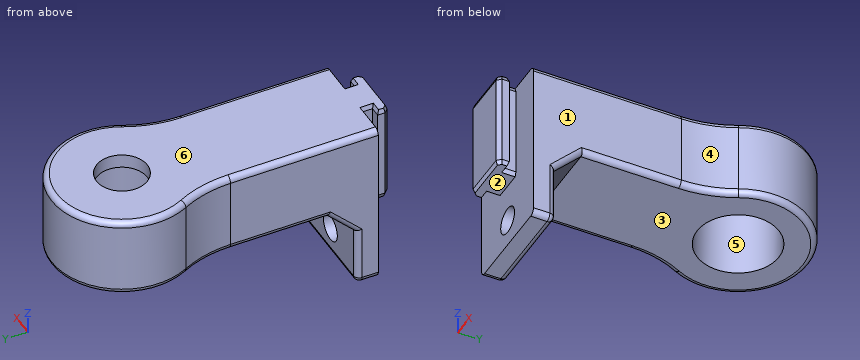
```python
from build123d import *
from OCP.BRepFilletAPI import BRepFilletAPI_MakeChamfer

# Parameters (mm, degrees)
SKETCH_1_R          = 4.5
EXTRUDE_1_DEPTH     = 2.5
EXTRUDE_START       = -12
SKETCH_1_13_R       = 7.25
SKETCH_1_13_R_2     = 4.5
EXTRUDE_5_DEPTH     = 12
EXTRUDE_START_2     = -7.5
EXTRUDE_2_DEPTH     = 20
EXTRUDE_3_DEPTH     = 15.5
SKETCH_4_R          = 2.4
CUT_EXTRUDE_3_DEPTH = 58.989223137
CUT_EXTRUDE_5_DEPTH = 0.1
CHAMFER_3_SIZE      = 0.8
CHAMFER_3_SIZE2     = 0.291176187
CHAMFER_4_SIZE      = 5
FILLET_1_R          = 1


with BuildPart() as part:
    # 草图1 → 凸台-拉伸1 (new body)
    with BuildSketch(Plane.XY):
        with BuildLine():
            Line((2.9, 10), (9, 10))
            Line((9, 10), (9, 36.328599249))
            ThreePointArc((9, 36.328599249), (9.545912037, 40.969554058), (11.153846154, 45.357153557))
            ThreePointArc((11.153846154, 45.357153557), (0, 63.5), (-11.153846154, 45.357153557))
            ThreePointArc((-11.153846154, 45.357153557), (-9.545912037, 40.969554058), (-9, 36.328599249))
            Line((-9, 36.328599249), (-9, 10))
            Line((-9, 10), (-2.9, 10))
            Line((-2.9, 10), (-2.9, 8))
            Line((-2.9, 8), (-4.7, 8))
            Line((-4.7, 8), (-4.7, 6.7))
            Line((-4.7, 6.7), (-4, 6))
            Line((-4, 6), (4, 6))
            Line((4, 6), (4.7, 6.7))
            Line((4.7, 6.7), (4.7, 8))
            Line((4.7, 8), (2.9, 8))
            Line((2.9, 8), (2.9, 10))
        make_face()
        with Locations((0, 51)):
            Circle(SKETCH_1_R, mode=Mode.SUBTRACT)
    extrude(amount=EXTRUDE_1_DEPTH)

    # 草图1<13> → 凸台-拉伸5 (add)
    # profile 1 of 4: a face of its own
    with BuildSketch(Plane.XY.offset(EXTRUDE_START)):
        Polygon((2.9, 10), (9, 10), (9, 14), (-9, 14), (-9, 10), (-2.9, 10), align=None)
    # profile 2 of 4: a face of its own
    with BuildSketch(Plane.XY.offset(EXTRUDE_START)):
        Polygon((2.9, 8), (2.9, 10), (-2.9, 10), (-2.9, 8), (-4.7, 8), (-4.7, 6.7), (-4, 6), (4, 6), (4.7, 6.7), (4.7, 8), align=None)
    # profile 3 of 4: a face of its own
    with BuildSketch(Plane.XY.offset(EXTRUDE_START)):
        with BuildLine():
            Line((-9, 14), (9, 14))
            Line((9, 14), (9, 36.328599249))
            ThreePointArc((9, 36.328599249), (9.545912037, 40.969554058), (11.153846154, 45.357153557))
            ThreePointArc((11.153846154, 45.357153557), (0, 63.5), (-11.153846154, 45.357153557))
            ThreePointArc((-11.153846154, 45.357153557), (-9.545912037, 40.969554058), (-9, 36.328599249))
            Line((-9, 36.328599249), (-9, 14))
        make_face()
        with Locations((0, 51)):
            Circle(SKETCH_1_13_R, mode=Mode.SUBTRACT)
    # profile 4 of 4: a face of its own
    with BuildSketch(Plane.XY.offset(EXTRUDE_START)):
        with Locations((0, 51)):
            Circle(SKETCH_1_13_R_2)
    extrude(amount=EXTRUDE_5_DEPTH)


with BuildPart() as extrude_5_kept_piece:
    # of the separate pieces the step leaves, the one the design keeps (extrude_5_pieces_kept)
    add(part.part.solids().sort_by_distance((2.9, 10, 2.5))[0])

    # 草图1<10> → 凸台-拉伸2 (add)
    with BuildSketch(Plane.XY.offset(EXTRUDE_START_2)):
        Polygon((2.9, 10), (9, 10), (9, 14), (-9, 14), (-9, 10), (-2.9, 10), align=None)
    extrude(amount=-EXTRUDE_2_DEPTH)

    # 草图1<11> → 凸台-拉伸3 (add)
    with BuildSketch(Plane.XY):
        Polygon((2.9, 8), (4.7, 8), (4.7, 6.7), (4, 6), (-4, 6), (-4.7, 6.7), (-4.7, 8), (-2.9, 8), (-2.9, 10), (2.9, 10), align=None)
    extrude(amount=-EXTRUDE_3_DEPTH)

    # 草图4 → 切除-拉伸3 (cut, through all)
    with BuildSketch(Plane(origin=(0, 14, 0), x_dir=(1, 0, 0), z_dir=(0, 1, 0))):
        with Locations(Location((0, 22.5, 0), (0, 0, 270))):
            Circle(SKETCH_4_R)
    extrude(amount=-CUT_EXTRUDE_3_DEPTH, mode=Mode.SUBTRACT)

    # 草图7 → 切除-拉伸5 (cut)
    with BuildSketch(Plane.XZ.offset(-10)):
        Polygon((2.9, 2.5), (9, 2.5), (9, -27.5), (-9, -27.5), (-9, 2.5), (-2.9, 2.5), (-2.9, -15.5), (2.9, -15.5), align=None)
    extrude(amount=-CUT_EXTRUDE_5_DEPTH, mode=Mode.SUBTRACT)

    # 倒角3: one chamfer whose edges measure the first distance from different faces: ONE call of the kernel's chamfer builder (chamfer() names one face for all edges)
    chamfer_3_edges_1 = [extrude_5_kept_piece.edges().sort_by_distance(p)[0] for p in [
        (2.9, 9.05, -15.5),
        (2.9, 9.05, 2.5),
    ]]
    chamfer_3_side_1 = [extrude_5_kept_piece.faces().sort_by_distance(p)[0] for p in [
        (2.9, 9.05, -6.5),
    ]]
    chamfer_3_edges_2 = [extrude_5_kept_piece.edges().sort_by_distance(p)[0] for p in [
        (4.7, 7.35, -15.5),
        (4.7, 7.35, 2.5),
    ]]
    chamfer_3_side_2 = [extrude_5_kept_piece.faces().sort_by_distance(p)[0] for p in [
        (4.7, 7.35, -6.5),
    ]]
    chamfer_3_edges_3 = [extrude_5_kept_piece.edges().sort_by_distance(p)[0] for p in [
        (4.35, 6.35, -15.5),
        (4.35, 6.35, 2.5),
    ]]
    chamfer_3_side_3 = [extrude_5_kept_piece.faces().sort_by_distance(p)[0] for p in [
        (4.35, 6.35, -6.5),
    ]]
    chamfer_3_edges_4 = [extrude_5_kept_piece.edges().sort_by_distance(p)[0] for p in [
        (3.8, 8, -15.5),
        (3.8, 8, 2.5),
    ]]
    chamfer_3_side_4 = [extrude_5_kept_piece.faces().sort_by_distance(p)[0] for p in [
        (3.8, 8, -6.5),
    ]]
    chamfer_3_edges_5 = [extrude_5_kept_piece.edges().sort_by_distance(p)[0] for p in [
        (0, 6, -15.5),
        (0, 6, 2.5),
    ]]
    chamfer_3_side_5 = [extrude_5_kept_piece.faces().sort_by_distance(p)[0] for p in [
        (0, 6, -6.5),
    ]]
    chamfer_3_edges_6 = [extrude_5_kept_piece.edges().sort_by_distance(p)[0] for p in [
        (-4.35, 6.35, -15.5),
        (-4.35, 6.35, 2.5),
    ]]
    chamfer_3_side_6 = [extrude_5_kept_piece.faces().sort_by_distance(p)[0] for p in [
        (-4.35, 6.35, -6.5),
    ]]
    chamfer_3_edges_7 = [extrude_5_kept_piece.edges().sort_by_distance(p)[0] for p in [
        (-4.7, 7.35, -15.5),
        (-4.7, 7.35, 2.5),
    ]]
    chamfer_3_side_7 = [extrude_5_kept_piece.faces().sort_by_distance(p)[0] for p in [
        (-4.7, 7.35, -6.5),
    ]]
    chamfer_3_edges_8 = [extrude_5_kept_piece.edges().sort_by_distance(p)[0] for p in [
        (-3.8, 8, -15.5),
        (-3.8, 8, 2.5),
    ]]
    chamfer_3_side_8 = [extrude_5_kept_piece.faces().sort_by_distance(p)[0] for p in [
        (-3.8, 8, -6.5),
    ]]
    chamfer_3_edges_9 = [extrude_5_kept_piece.edges().sort_by_distance(p)[0] for p in [
        (-2.9, 9.05, -15.5),
        (-2.9, 9.05, 2.5),
    ]]
    chamfer_3_side_9 = [extrude_5_kept_piece.faces().sort_by_distance(p)[0] for p in [
        (-2.9, 9.05, -6.5),
    ]]
    chamfer_3 = BRepFilletAPI_MakeChamfer(extrude_5_kept_piece.part.solid().wrapped)
    for e in chamfer_3_edges_1:
        chamfer_3.Add(CHAMFER_3_SIZE, CHAMFER_3_SIZE2, e.wrapped, chamfer_3_side_1[0].wrapped)  # the first distance lies on this face
    for e in chamfer_3_edges_2:
        chamfer_3.Add(CHAMFER_3_SIZE, CHAMFER_3_SIZE2, e.wrapped, chamfer_3_side_2[0].wrapped)  # the first distance lies on this face
    for e in chamfer_3_edges_3:
        chamfer_3.Add(CHAMFER_3_SIZE, CHAMFER_3_SIZE2, e.wrapped, chamfer_3_side_3[0].wrapped)  # the first distance lies on this face
    for e in chamfer_3_edges_4:
        chamfer_3.Add(CHAMFER_3_SIZE, CHAMFER_3_SIZE2, e.wrapped, chamfer_3_side_4[0].wrapped)  # the first distance lies on this face
    for e in chamfer_3_edges_5:
        chamfer_3.Add(CHAMFER_3_SIZE, CHAMFER_3_SIZE2, e.wrapped, chamfer_3_side_5[0].wrapped)  # the first distance lies on this face
    for e in chamfer_3_edges_6:
        chamfer_3.Add(CHAMFER_3_SIZE, CHAMFER_3_SIZE2, e.wrapped, chamfer_3_side_6[0].wrapped)  # the first distance lies on this face
    for e in chamfer_3_edges_7:
        chamfer_3.Add(CHAMFER_3_SIZE, CHAMFER_3_SIZE2, e.wrapped, chamfer_3_side_7[0].wrapped)  # the first distance lies on this face
    for e in chamfer_3_edges_8:
        chamfer_3.Add(CHAMFER_3_SIZE, CHAMFER_3_SIZE2, e.wrapped, chamfer_3_side_8[0].wrapped)  # the first distance lies on this face
    for e in chamfer_3_edges_9:
        chamfer_3.Add(CHAMFER_3_SIZE, CHAMFER_3_SIZE2, e.wrapped, chamfer_3_side_9[0].wrapped)  # the first distance lies on this face
    add(Compound.cast(chamfer_3.Shape()), mode=Mode.REPLACE)

    # 倒角4
    chamfer_4_edges = [extrude_5_kept_piece.edges().sort_by_distance(p)[0] for p in [
        (0, 14, -12),
    ]]
    chamfer(chamfer_4_edges, length=CHAMFER_4_SIZE)

    # 圆角1
    fillet_1_edges = [extrude_5_kept_piece.edges().sort_by_distance(p)[0] for p in [
        (-9, 14, -22.25),
        (9, 14, -22.25),
        (0, 14, -27.5),
        (-9, 12.05, -27.5),
        (9, 12.05, -27.5),
        (9, 23.214299624, 2.5),
        (-9, 23.214299624, 2.5),
        (9.545912037, 40.969554058, 2.5),
        (0, 63.5, 2.5),
        (-9, 27.664299624, -12),
        (9, 27.664299624, -12),
        (9, 16.5, -14.5),
        (-9, 16.5, -14.5),
        (-9.545912037, 40.969554058, 2.5),
        (0, 63.5, -12),
        (9.545912037, 40.969554058, -12),
        (-9.545912037, 40.969554058, -12),
    ]]
    fillet(fillet_1_edges, radius=FILLET_1_R)


solid = extrude_5_kept_piece.part
```
Geometry check sheet. Reference: the model listing, model coordinates, mm. Face numbers are marked on the shaded views. A direction names the side the tool comes from. Coordinates: 2 decimals unless noted, no trailing zeros. Order: outer loops, then holes, each group sorted by start corner. A loop starts at its lowest first (then second) coordinate and runs counter-clockwise, first axis right, second up.
Item 1: Section check C-C (y = 24.5). Enter the section's corners in (x, z), plus the area to 3 significant figures.
Item 2: Scan lines: line 1 along Y through (x, z) = (0, 1.3); line 2 along X through (y, z) = (12.7, -22.5); line 3 along Y through (x, z) = (0, -3). Record each from-to range of solid material in increasing order.
Item 3: Depth check by flat-ended pin: pin 1 (13 mm diameter, centred on y = 20, z = -18, fed in from -X); pin 2 (1.4 mm diameter, centred on y = 7, z = -9, fed in from -X); pin 3 (5 mm diameter, centred on x = 3, y = 29, fed in from -Z). Enter the tip coordinate at first touch or a pass-through.
Item 4: Tool access check on the marked faces 1, 2 and 3. Record the directions out of +Z, -Z, +X, -X, +Y, -Y that give a thin tool (end or side, any length) a straight path to the whole face; none if there is none.
Item 5: Section check B-B (x = 0). Enter the section's corners in (y, z), plus the area to 3 significant figures.
Item 6: Section check D-D (z = -8.25). Enter the section's corners in (x, y).
Item 7: Section check A-A (z = -22.5). Enter the section's corners in (x, y), plus the area to 3 significant figures.
Item 8: Mould release check, pull along Y, two halves, no side actions. Record for the marked faces 4, 5 and 6: released by +Y, released by -Y, zero draft, split by the parting line, or undercut.
Check sheet entries:
1. outline: (-9, -11) arc R1 ccw to (-8, -12) - (8, -12) arc R1 ccw to (9, -11) - (9, 1.5) arc R1 ccw to (8, 2.5) - (-8, 2.5) arc R1 ccw to (-9, 1.5) - close
1. area: 260 mm2
2. line 1: y = 6 to 46.5, 55.5 to 63.5
2. line 2: x = -9 to -2.4, 2.4 to 9
2. line 3: y = 6 to 43.75, 58.25 to 63.5
3. pin 1: stops at x = -9
3. pin 2: stops at x = -4.7
3. pin 3: stops at z = -12
4. face 1: +Z, -Z, +X, -Y
4. face 2: -Z, +X, -X, -Y
4. face 3: -Z, +X, -X, +Y
5. outline: (6, -14.7) - (6.29, -15.5) - (10.1, -15.5) - (10.1, -20.1) - (14, -20.1) - (14, -17) - (19, -12) - (43.75, -12) - (43.75, 0) - (46.5, 0) - (46.5, 2.5) - (6.29, 2.5) - (6, 1.7) - close; (10.1, -27.5) - (13, -27.5) arc R1 ccw to (14, -26.5) - (14, -24.9) - (10.1, -24.9) - close; (55.5, 0) - (58.25, 0) - (58.25, -12) - (62.5, -12) arc R1 ccw to (63.5, -11) - (63.5, 1.5) arc R1 ccw to (62.5, 2.5) - (55.5, 2.5) - close
5. area: 705 mm2
6. outline: (-11.15, 45.36) arc R20 cw to (-9, 36.33) - (-9, 10.1) - (-2.9, 10.1) - (-2.9, 8) - (-4.7, 8) - (-4.7, 6.7) - (-4, 6) - (4, 6) - (4.7, 6.7) - (4.7, 8) - (2.9, 8) - (2.9, 10.1) - (9, 10.1) - (9, 36.33) arc R20 cw to (11.15, 45.36) arc R12.5 ccw (long way) to start; hole circle Ø14.5 at (0, 51)
7. outline: (-9, 10.1) - (-2.4, 10.1) - (-2.4, 14) - (-8, 14) arc R1 ccw to (-9, 13) - close; (2.4, 10.1) - (9, 10.1) - (9, 13) arc R1 ccw to (8, 14) - (2.4, 14) - close
7. area: 51.1 mm2
8. face 4: released by -Y
8. face 5: undercut
8. face 6: zero draft
